```python
from build123d import *

# Parameters (mm, degrees)
FILLET_R            = 1
SKETCH001_R         = 15.5
SKETCH001_R_2       = 13.5
PAD_DEPTH           = 1
LINEARPATTERN_COUNT = 35
LINEARPATTERN_PITCH = 3.911765


with BuildPart() as part:
    # Sketch → Revolution (revolve)
    with BuildSketch(Plane.XZ):
        Polygon((140, 0), (137, 0), (137, 10.5), (0, 10.5), (0, 25), (5, 25), (5, 13.5), (140, 13.5), align=None)
    revolve(axis=Axis((0, 0, 0), (1, 0, 0)))

    # Fillet
    fillet_edges = [part.edges().sort_by_distance(p)[0] for p in [
        (0, 0, -25),
        (5, 0, -25),
        (2.5, 0, 25),
    ]]
    fillet(fillet_edges, radius=FILLET_R)

    # Sketch001 (on Face9 of Fillet) → Pad (new body, symmetric)
    with BuildSketch(Plane(origin=(140, 0, 0), x_dir=(0, 0, 1), z_dir=(1, 0, 0))):
        Circle(SKETCH001_R)
        Circle(SKETCH001_R_2, mode=Mode.SUBTRACT)
    pad = extrude(amount=PAD_DEPTH, both=True)

    # LinearPattern: Pad ×35
    with Locations(*[(-i * LINEARPATTERN_PITCH, 0, 0) for i in range(1, LINEARPATTERN_COUNT)]):
        add(pad)


solid = part.part
```
Check sheet for the modelled part. Datum: model origin and axes. Units: mm. A direction names the side the tool comes from. Round coordinates to 2 decimals unless told otherwise and drop trailing zeros.
1) Go/stop test with flat-tipped pins: pin 1 Ø2 at (x, y) = (91.5, -10) entering from +Z; pin 2 Ø9.5 at (y, z) = (-6.5, 0) entering from +X; pin 3 Ø5 at (x, y) = (94, 13.5) entering from +Z. Record where each tip stops, or that it passes through.
2) Scan lines: line 1 (Z direction, x = 106, y = 0); line 2 (Y direction, x = 140.3, z = 0). Record each from-to range of solid material in increasing order.
3) Mould release check, pull along X, two halves, no side actions. Record for faces 1 (the cylindrical face through (83.29, 13.18, -2.93)), 2 (the cylindrical face through (53.955, -15.368, -2.018)): +X half, -X half, draft (parallel to the pull), parting line (faces both ways), or undercut.
4) Tool access check on faces 3 (the flat face through (58.853, -13, -5)), 4 (the cylindrical face through (85.249, -15.368, -2.018)). Record the directions out of +Z, -Z, +X, -X, +Y, -Y that give a thin tool (end or side, any length) a straight path to the whole face; none if there is none.
Result:
1. pin 1: stops at z = 12.5
1. pin 2: stops at x = 140
1. pin 3: stops at z = 10.92
2. line 1: z = -13.5 to -10.5, 10.5 to 13.5
2. line 2: y = -15.5 to -13.5, 13.5 to 15.5
3. face 1: undercut
3. face 2: draft
4. face 3: none
4. face 4: +X
